Here's how the part is built. I have some questions about the finished solid (model axes, mm). Face numbers are marked on the shaded views. Coordinates: 2 decimals unless noted, no trailing zeros. Loops run counter-clockwise (first coordinate to the right, second up) from the corner with the lowest first, then second, coordinate; pieces in that order, holes last. Notation, with made-up numbers: (-1, -21) - (43, -21) arc R21 ccw to (43, -5) - close; hole circle Ø9 at (-35.5, 81.25). An arc over 180 degrees is marked (long way). Use a Markdown table: item, result.
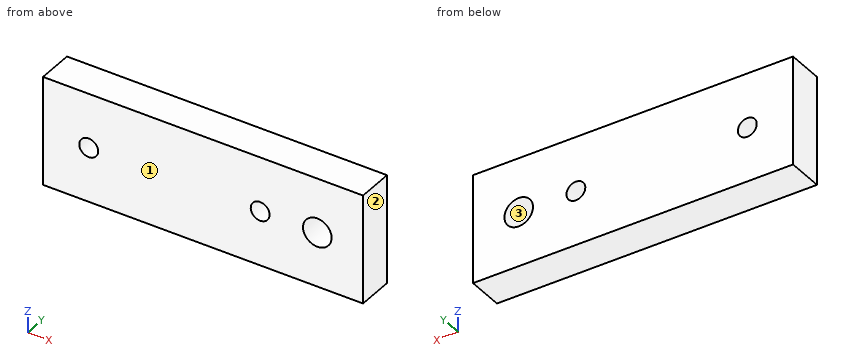
```python
from build123d import *

# Parameters (mm, degrees)
SKETCH1_W             = 56
SKETCH1_H             = 19.05
BOSS_EXTRUDE1_DEPTH   = 6.35
M6X1_0_TAPPED_HOLE1_D = 5
M4X0_7_TAPPED_HOLE1_D = 3.3


with BuildPart() as part:
    # Sketch1 → Boss-Extrude1 (new body)
    with BuildSketch(Plane(origin=(0, 0, 0), x_dir=(1, 0, 0), z_dir=(0, 1, 0))):
        Rectangle(SKETCH1_W, SKETCH1_H)
    extrude(amount=BOSS_EXTRUDE1_DEPTH)

    # M6x1.0 Tapped Hole1 (through all)
    with Locations(Plane(origin=(20, 6.35, 0), x_dir=(0, 0, 1), z_dir=(0, 1, 0))):
        with Locations((0, 0)):
            Hole(M6X1_0_TAPPED_HOLE1_D / 2)

    # M4x0.7 Tapped Hole1 (through all)
    with Locations(Plane(origin=(-20, 6.35, 0), x_dir=(0, 0, 1), z_dir=(0, 1, 0))):
        with Locations((0, 0), (0, 30)):
            Hole(M4X0_7_TAPPED_HOLE1_D / 2)


solid = part.part
```
Q1. I want a section at B-B, the plane x = 20. Write out the boundary of the cut face in (y, z) (3 decimals), then the cut area to 3 significant figures.
Check values:
| item | result |
|---|---|
| outline | (0, -9.525) - (6.35, -9.525) - (6.35, -2.5) - (0, -2.5) - close; (0, 2.5) - (6.35, 2.5) - (6.35, 9.525) - (0, 9.525) - close |
| area | 89.2 mm^2 |
Q2. I want a section at C-C, the plane y = 1. Write out the boundary of the cut face in (x, z) (3 decimals).
Check values:
| item | result |
|---|---|
| outline | (-28, -9.525) - (28, -9.525) - (28, 9.525) - (-28, 9.525) - close; hole circle Ø3.3 at (-20, 0); hole circle Ø3.3 at (10, 0); hole circle Ø5 at (20, 0) |
Q3. I want a section at A-A, the plane z = 0. Write out the boundary of the cut face in (x, y).
Check values:
| item | result |
|---|---|
| outline | (-28, 0) - (-21.65, 0) - (-21.65, 6.35) - (-28, 6.35) - close; (-18.35, 0) - (8.35, 0) - (8.35, 6.35) - (-18.35, 6.35) - close; (11.65, 0) - (17.5, 0) - (17.5, 6.35) - (11.65, 6.35) - close; (22.5, 0) - (28, 0) - (28, 6.35) - (22.5, 6.35) - close |
Q4. I want a section at D-D, the plane x = -20. Write out the boundary of the cut face in (y, z) (3 decimals), then the cut area to 3 significant figures.
Check values:
| item | result |
|---|---|
| outline | (0, -9.525) - (6.35, -9.525) - (6.35, -1.65) - (0, -1.65) - close; (0, 1.65) - (6.35, 1.65) - (6.35, 9.525) - (0, 9.525) - close |
| area | 100 mm^2 |
Q5. Please list where these lines run through material, in increasing order: L1, parallel to X at y = 4.25, z = 0; L2, parallel to X at y = 4.75, z = 1; L3, parallel to Z at x = 8.5, y = 1 (3 decimals). Write a range as from..to.
Check values:
| item | result |
|---|---|
| L1 | -28..-21.65, -18.35..8.35, 11.65..17.5, 22.5..28 |
| L2 | -28..-21.31, -18.69..8.69, 11.31..17.71, 22.29..28 |
| L3 | -9.525..-0.687, 0.687..9.525 |
Q6. If we mould it in two halves opening along X, with no side actions, what happens to the marked faces 1, 2 and 3? For each: pulls with the +X half, pulls with the -X half, needs draft (parallel to the pull), parting line crosses it, or undercut.
Check values:
| item | result |
|---|---|
| face 1 | needs draft |
| face 2 | pulls with the +X half |
| face 3 | undercut |
